Can you work these out from the drawing? Everything is in mm from the part's minimum corner. A direction names the side the tool comes from. Round coordinates to 2 decimals unless told otherwise and drop trailing zeros. Order: outer loops, then holes, each group sorted by start corner. A loop starts at its lowest first (then second) coordinate and runs counter-clockwise, first axis right, second up. Notation, with made-up numbers: (53.25, 66) -> (109.25, 66) arc R17 cw to (109.25, 73) -> close; hole circle Ø8 at (37.25, 58.5). An arc over 180 degrees is marked (long way). One line per item, written item: value.
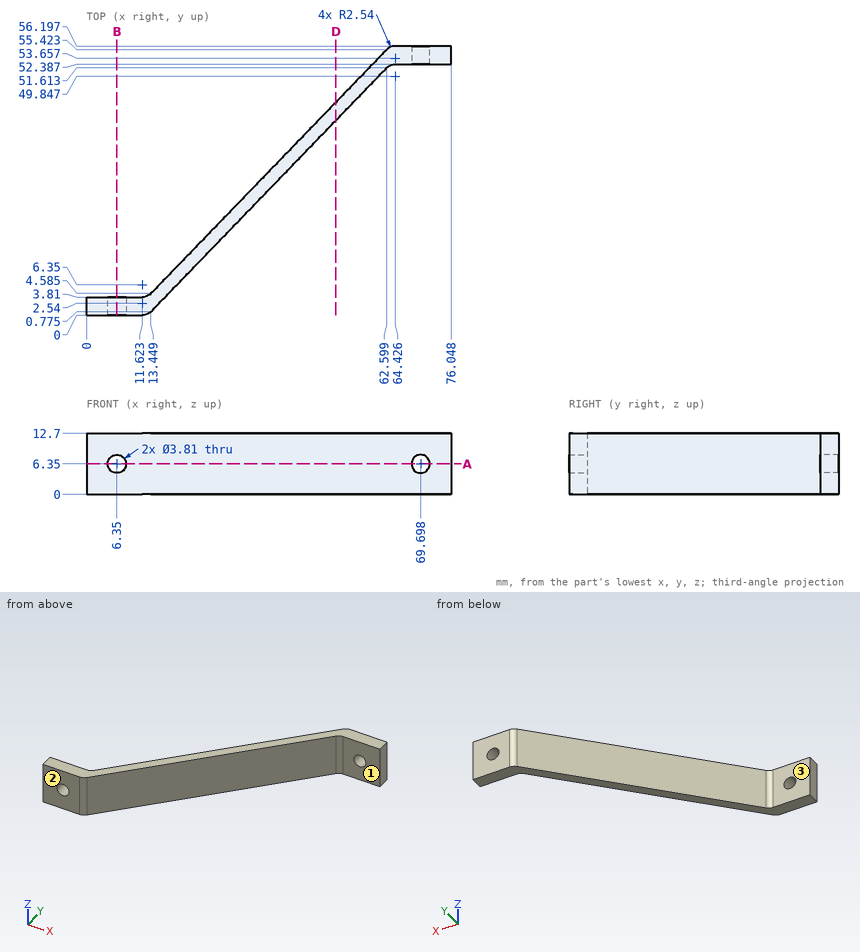
Q1. I want a section at B-B on x = 6.35. List the corners of the cut face in (y, z) for me (1 decimal).
Answers below:
outline: (0, 0) -> (3.8, 0) -> (3.8, 4.4) -> (0, 4.4) -> close; (0, 8.3) -> (3.8, 8.3) -> (3.8, 12.7) -> (0, 12.7) -> close
Q2. Please list where these lines run through material, in increasing order: line 1 along X through (y, z) = (1.6, 6.35) (1 decimal); line 2 along Z through (x, y) = (6, 2); line 3 along X through (y, z) = (1.95, 6.35) (1 decimal).
Answers below:
line 1: 0 to 4.4, 8.3 to 14.2
line 2: 0 to 4.48, 8.22 to 12.7
line 3: 0 to 4.4, 8.3 to 14.6
Q3. On a 3-axis mill with a long thin cutter (end or side, diameter ignored), from which of +Z, -Z, +X, -X, +Y, -Y can I reach the whole of each face in a straight line? I mean the marked faces 1, 2 and 3. Say none if no direction works.
Answers below:
face 1: +Z, -Z, +X, -Y
face 2: +Z, -Z, +X, -X, -Y
face 3: +Z, -Z, -X, +Y
Q4. Will these pins go through, and if not, where does the flat tip stop? pin 1 Ø4 at (x, z) = (32.5, 1.5) entering from -Y; pin 2 Ø1 at (y, z) = (33, 1.5) entering from -X; pin 3 Ø6 at (x, z) = (4.5, 6.5) entering from +Y; pin 4 Ø1.5 at (x, y) = (25, 17) entering from -Z.
Answers below:
pin 1: y = 18.41
pin 2: x = 40.44
pin 3: y = 3.81
pin 4: z = 0
Q5. I want a section at A-A on z = 6.35. Give the number of separate pieces and of enclosed holes in the cut face, plus the area to 3 significant figures.
Answers below:
separate pieces: 3
enclosed holes: 0
area: 261 mm^2
Q6. I want a section at D-D on x = 52. List the corners of the cut face in (y, z) for me.
Answers below:
outline: (40.65, 0) -> (44.46, 0) -> (44.46, 12.7) -> (40.65, 12.7) -> close
